Autodesk Inventor part; units mm, degrees
ref_plane "YZ Plane" through (0, 0, 0) normal (1, 0, 0) x (0, 1, 0)
ref_plane "XZ Plane" through (0, 0, 0) normal (0, 1, 0) x (-1, 0, 0)
ref_plane "XY Plane" through (0, 0, 0) normal (0, 0, 1) x (1, 0, 0)
sketch "Boceto1" plane through (0, 0, 0) normal (0, 1, 0) x (-1, 0, 0)
  line L0 (44, 22.5) -> (-44, 22.5)
  line L1 (-44, 22.5) -> (-44, -22.5)
  line L2 (-44, -22.5) -> (44, -22.5)
  line L3 (44, -22.5) -> (44, 22.5)
  line L4 (44, 22.5) -> (-44, -22.5) construction
  circle A0 centre (14.75, -16.5) radius 2.5
  circle A1 centre (14.75, 9.2) radius 2.5
  line L5 (14.75, -16.5) -> (-14.75, -16.5) construction
  line L6 (-14.75, -16.5) -> (-14.75, 9.2) construction
  line L7 (-14.75, 9.2) -> (14.75, 9.2) construction
  line L8 (14.75, 9.2) -> (14.75, -16.5) construction
  line L9 (0, 0) -> (0, -30.1177)
  circle A2 centre (-14.75, -16.5) radius 2.5
  circle A3 centre (-14.75, 9.2) radius 2.5
  dimension "d0" = 88
  dimension "d1" = 45
  dimension "d4" = 5
  dimension "d5" = 25.7
  dimension "d6" = 6
  dimension "d7" = 29.5
extrude "Extrusión1" add sketch "Boceto1" along normal blind 2
properties part number "PlacaSTC-HH20"
Here's how the part is built. I have some questions about the finished solid (model axes, mm). Coordinates: 2 decimals unless noted, no trailing zeros. Loops run counter-clockwise (first coordinate to the right, second up) from the corner with the lowest first, then second, coordinate; pieces in that order, holes last. Notation, with made-up numbers: (69, 45) -> (89, 45) arc R15 cw to (89, 50) -> close; hole circle Ø9 at (20, 85.5). An arc over 180 degrees is marked (long way). Return JSON: item names as keys, results as strings.
1) Thinking about a two-plate mould opening in X: for faces 1 (the face through (17.248, 0.986, -16.61)), 2 (the face through (-44, 1, 0)), 3 (the face through (1, 1, -22.5)), which applies, +X half, -X half, draft (parallel to the pull), parting line (faces both ways), or undercut?
Results below:
{"face 1": "undercut", "face 2": "-X half", "face 3": "draft"}
2) If we section it at B-B, the plane x = 14.75: Write out the boundary of the cut face in (y, z).
Results below:
{"outline": "(0, -22.5) -> (2, -22.5) -> (2, -19) -> (0, -19) -> close; (0, -14) -> (2, -14) -> (2, 6.7) -> (0, 6.7) -> close; (0, 11.7) -> (2, 11.7) -> (2, 22.5) -> (0, 22.5) -> close"}
3) If we section it at A-A, the plane z = -16.5: Write out the boundary of the cut face in (x, y).
Results below:
{"outline": "(-44, 0) -> (-17.25, 0) -> (-17.25, 2) -> (-44, 2) -> close; (-12.25, 0) -> (12.25, 0) -> (12.25, 2) -> (-12.25, 2) -> close; (17.25, 0) -> (44, 0) -> (44, 2) -> (17.25, 2) -> close"}
4) If we section it at C-C, the plane y = 1.55: Write out the boundary of the cut face in (x, z).
Results below:
{"outline": "(-44, -22.5) -> (44, -22.5) -> (44, 22.5) -> (-44, 22.5) -> close; hole circle Ø5 at (-14.75, -16.5); hole circle Ø5 at (-14.75, 9.2); hole circle Ø5 at (14.75, -16.5); hole circle Ø5 at (14.75, 9.2)"}
5) I need wall thicknesses on line 1 (Z direction, x = -14.5, y = 0.95); line 2 (Z direction, x = -16, y = 1.2). Which ranges of each line are inside material? Lowest first, please. Write a range as from..to.
Results below:
{"line 1": "-22.5..-18.99, -14.01..6.71, 11.69..22.5", "line 2": "-22.5..-18.67, -14.33..7.03, 11.37..22.5"}
6) Will this pin go through, and if not, where does the flat tip stop? pin 1 (4.5 mm diameter, centred on x = -14.75, z = 9.2, fed in from +Y).
Results below:
{"pin 1": "through"}
